Check sheet for the modelled part. Datum: model origin and axes. Units: mm. Round coordinates to 2 decimals unless told otherwise and drop trailing zeros. Write each loop counter-clockwise with the first axis right and the second up, starting at its lowest first coordinate (ties: lowest second). Pieces come first, ordered by that corner, then holes.
Item 1: Section check C-C, the plane y = -0.5. Record the cut outline in (x, z).
Item 2: Material ranges on line 1 along Y through (x, z) = (10, 78); line 2 along Y through (x, z) = (37, 1912); line 3 along X through (y, z) = (-23, 1862.5), recorded low to high.
Item 3: Depth check by flat-ended pin: pin 1 (14 mm diameter, centred on y = -4, z = 766, fed in from +X); pin 2 (8 mm diameter, centred on x = 4, y = 25.5, fed in from +Z). Enter the tip coordinate at first touch or a pass-through.
Item 4: Section check B-B, the plane z = 558.5. Record the cut outline in (x, y), plus the area to 3 significant figures.
Item 5: Section check A-A, the plane x = 31. Record the cut outline in (y, z), plus the area to 3 significant figures.
Item 6: Release check for a two-part mould opening along Y. For faces 1 (the flat face through (3, 0, 0)), 2 (the flat face through (-1.43, -1, 1185)), 3 (the flat face through (21, -40, 1185)), 4 (the flat face through (4.07, 0, 1185)) record: pulls with the +Y half, pulls with the -Y half, needs draft (parallel to the pull), parting line crosses it, or undercut.
Autodesk Inventor part; units mm, degrees
ref_plane "Начальная плоскость" through (0, 0, -40) normal (0, 0, 1) x (1, 0, 0)
ref_plane "Конечная плоскость" through (0, 0, 2445) normal (0, 0, 1) x (1, 0, 0)
ref_plane "РабПлоскость4" through (21.07, -40, -40) normal (0, 0.7071, -0.7071) x (1, 0, 0)
ref_plane "Начальная плоскость" through (0, 0, -40) normal (0, 0, 1) x (1, 0, 0)
ref_plane "Конечная плоскость" through (0, 0, 2445) normal (0, 0, 1) x (1, 0, 0)
sketch "Эскиз" plane through (0, 0, 0) normal (0, 0, 1) x (1, 0, 0)
  line L0 (-1.43, 0) -> (-1.43, 40)
  line L1 (-1.43, 40) -> (43.57, 40)
  line L2 (43.57, 40) -> (43.57, 38.1774)
  line L3 (39.9881, 34.1993) -> (11.2338, 31.1771)
  line L4 (4.07, 23.221) -> (4.07, 0)
  line L5 (4.07, 0) -> (-1.43, 0) construction
  line L6 (23.82, 40) -> (23.82, 32.5) construction
  line L7 (43.57, 34.5758) -> (43.57, 32.5) construction
  line L8 (43.57, 32.5) -> (23.82, 32.5) construction
  line L9 (0, 15) -> (0, -27) construction
  line L10 (-5.539, 0) -> (16.0067, 0) construction
  line L11 (-1.43, 0) -> (-1.43, -40)
  line L12 (-1.43, -40) -> (43.57, -40)
  line L13 (43.57, -40) -> (43.57, -38.1774)
  line L14 (39.9881, -34.1993) -> (11.2338, -31.1771)
  line L15 (4.07, -23.221) -> (4.07, 0)
  arc A0 (11.2338, 31.1771) -> (4.07, 23.221) centre (12.07, 23.221) ccw
  arc A1 (4.07, -23.221) -> (11.2338, -31.1771) centre (12.07, -23.221) ccw
  arc A2 (39.9881, 34.1993) -> (43.57, 38.1774) centre (39.57, 38.1774) ccw
  arc A3 (43.57, -38.1774) -> (39.9881, -34.1993) centre (39.57, -38.1774) ccw
  line L16 (0, 56) -> (0, -56) construction
  line L17 (-15.5135, 0) -> (54.308, 0) construction
  point P0 (4.07, 30.4242)
  point P1 (43.57, -34.5758)
  point P2 (4.07, -30.4242)
  point P3 (23.82, -40)
  point P4 (23.82, -32.5)
  dimension "d0" = 5.5
  dimension "d1" = 40
  dimension "d2" = 45
  dimension "d3" = 7.5
  dimension "d4" = 19.75
  dimension "d5" = 2.0758
  dimension "d23" = 8
  dimension "d24" = 4
  dimension "d25" = 1.43
extrude "Тело" add sketch "Эскиз" along normal up to surface (2485 mm away) from surface at -40
sketch "Sketch3" plane through (0, 0, 0) normal (0, 0, 1) x (1, 0, 0)
  line L0 (0, 0) -> (10, 0)
ref_plane "Work Plane3" through (0, 0, 0) normal (0, -1, 0) x (1, 0, 0)
sketch "Sketch4" plane through (0, 0, 0) normal (0, -1, 0) x (1, 0, 0)
  line L0 (-2, -40) -> (12, -40)
  line L1 (-2, 2445) -> (12, 2445)
  dimension "d29" = 2485
ref_plane "РабПлоскость4" through (21.07, -40, -40) normal (0, 0.7071, -0.7071) x (1, 0, 0)
split "Разделение1" plane through (21.07, -40, -40) removes the side toward (0, 0.7071, -0.7071)
ref_plane "РабПлоскость5" through (21.07, -40, 2445) normal (0, 0.7071, 0.7071) x (1, 0, 0)
split "Разделение2" plane through (21.07, -40, 2445) removes the side toward (0, 0.7071, 0.7071)
equation "\"d0\" = G_T"
equation "\"d1\" = 0.5 * G_H"
equation "\"d2\" = G_W"
equation "\"d3\" = G_T1"
equation "\"d4\" = G_C"
equation "\"d23\" = G_IR"
equation "\"d24\" = G_ER"
equation "\"d25\" = ex"
equation "\"d6\" = G_L"
equation "\"G_W\" = 45"
equation "\"G_T\" = 5.5"
equation "\"G_T1\" = 7.5"
equation "\"G_NG\" = 0.105104"
equation "\"G_ER\" = 4"
equation "\"G_IR\" = 8"
equation "\"G_C\" = 19.75"
equation "\"G_L\" = d29"
equation "\"ex\" = 1.43"
equation "\"d27\" = G_OFFSET_END + B_L"
equation "\"B_L\" = 2405"
properties part number "ISO 657/11 - CH 80 x 8 - 2485" material "Сталь, мягкая"
Values found:
1. outline: (-1.43, -0.5) - (4.07, -0.5) - (4.07, 2405.5) - (-1.43, 2405.5) - close
2. line 1: y = -40 to -30.95, 30.95 to 40
2. line 2: y = -40 to -33.89, 33.89 to 40
2. line 3: x = -1.43 to 4.07
3. pin 1: stops at x = 4.07
3. pin 2: stops at z = 2383.5
4. outline: (-1.43, -40) - (43.57, -40) - (43.57, -38.18) arc R4 ccw to (39.99, -34.2) - (11.23, -31.18) arc R8 cw to (4.07, -23.22) - (4.07, 23.22) arc R8 cw to (11.23, 31.18) - (39.99, 34.2) arc R4 ccw to (43.57, 38.18) - (43.57, 40) - (-1.43, 40) - close
4. area: 1,050 mm2
5. outline: (-40, -40) - (-33.25, -33.25) - (-33.25, 2438.25) - (-40, 2445) - close; (33.25, 33.25) - (40, 40) - (40, 2365) - (33.25, 2371.75) - close
5. area: 32,400 mm2
6. face 1: pulls with the +Y half
6. face 2: needs draft
6. face 3: pulls with the -Y half
6. face 4: undercut
